```python
from build123d import *

# Parameters (mm, degrees)
SKETCH1_W           = 59.69
SKETCH1_H           = 25.4
BOSS_EXTRUDE1_DEPTH = 25.4
SKETCH2_W           = 15.24
SKETCH2_H           = 25.4
CUT_EXTRUDE1_DEPTH  = 19.05
SKETCH3_R           = 3.175
CUT_EXTRUDE2_DEPTH  = 67.101029493
SKETCH5_W           = 110.49
SKETCH5_H           = 25.4
BOSS_EXTRUDE2_DEPTH = 7.62
CUT_EXTRUDE4_DEPTH  = 92.095392309
CUT_EXTRUDE5_DEPTH  = 70.191693408
FILLET2_R           = 5.08
FILLET3_R           = 2.54


with BuildPart() as part:
    # Sketch1 → Boss-Extrude1 (new body)
    with BuildSketch(Plane(origin=(0, 0, 0), x_dir=(1, 0, 0), z_dir=(0, 1, 0))):
        Rectangle(SKETCH1_W, SKETCH1_H)
    extrude(amount=BOSS_EXTRUDE1_DEPTH)

    # Sketch2 → Cut-Extrude1 (cut)
    with BuildSketch(Plane(origin=(0, 25.4, 0), x_dir=(1, 0, 0), z_dir=(0, 1, 0))):
        Rectangle(SKETCH2_W, SKETCH2_H)
    extrude(amount=-CUT_EXTRUDE1_DEPTH, mode=Mode.SUBTRACT)

    # Sketch3 → Cut-Extrude2 (cut, through all)
    with BuildSketch(Plane.ZY.offset(29.845)):
        with Locations((0, 17.78)):
            Circle(SKETCH3_R)
    extrude(amount=-CUT_EXTRUDE2_DEPTH, mode=Mode.SUBTRACT)

    # Sketch5 → Boss-Extrude2 (add)
    with BuildSketch(Plane(origin=(0, 0, -12.7), x_dir=(-1, 0, 0), z_dir=(0, 0, -1))):
        with Locations((0, 12.7)):
            Rectangle(SKETCH5_W, SKETCH5_H)
    extrude(amount=BOSS_EXTRUDE2_DEPTH)

    # Sketch4 → Cut-Extrude4 (cut, through all)
    with BuildSketch(Plane(origin=(29.845, 0, 0), x_dir=(0, 0, -1), z_dir=(1, 0, 0))):
        with BuildLine():
            Line((-12.7, 6.35), (-12.7, 25.4))
            Line((-12.7, 25.4), (0, 25.4))
            add(Edge.make_bspline(
                [(-12.7, 6.35), (-6.35, 25.4), (0, 25.4)],
                knots=[0, 0, 0, 0.5, 0.5, 0.5], degree=2))
        make_face()
    extrude(amount=-CUT_EXTRUDE4_DEPTH, mode=Mode.SUBTRACT)

    # Sketch6 → Cut-Extrude5 (cut, through all)
    with BuildSketch(Plane(origin=(0, 0, -20.32), x_dir=(-1, 0, 0), z_dir=(0, 0, -1))):
        with BuildLine():
            Line((-44.37743079, 17.921542216), (-35.56, 17.921542216))
            ThreePointArc((-35.56, 17.921542216), (-29.939868166, 14.732), (-35.56, 11.542457784))
            Line((-35.56, 11.542457784), (-44.37743079, 11.542457784))
            ThreePointArc((-44.37743079, 11.542457784), (-47.566973006, 14.732), (-44.37743079, 17.921542216))
        make_face()
        with BuildLine():
            Line((35.56, 17.994815174), (45.556129925, 17.994815174))
            ThreePointArc((45.556129925, 17.994815174), (48.818945099, 14.732), (45.556129925, 11.469184826))
            Line((45.556129925, 11.469184826), (35.56, 11.469184826))
            ThreePointArc((35.56, 11.469184826), (29.876774509, 14.732), (35.56, 17.994815174))
        make_face()
    extrude(amount=-CUT_EXTRUDE5_DEPTH, mode=Mode.SUBTRACT)

    # Fillet2
    fillet2_edges = [part.edges().sort_by_distance(p)[0] for p in [
        (42.545, 0, -12.7),
        (-42.545, 0, -12.7),
        (29.845, 0, 0),
        (-29.845, 0, 0),
    ]]
    fillet(fillet2_edges, radius=FILLET2_R)

    # Fillet3
    fillet3_edges = [part.edges().sort_by_distance(p)[0] for p in [
        (0, 6.35, -12.7),
    ]]
    fillet(fillet3_edges, radius=FILLET3_R)


solid = part.part
```
The listing builds one solid part. Answer for the finished solid, in the listing's coordinates (mm). A direction names the side the tool comes from. Give positions to 0.01 mm unless a question says otherwise; leave off trailing zeros. Write each loop counter-clockwise with the first axis right and the second up, starting at its lowest first coordinate (ties: lowest second). Pieces come first, ordered by that corner, then holes. Notation, with made-up numbers: (60, 66) -> (101, 66) arc R15 cw to (101, 70) -> close; hole circle Ø2 at (14.5, 63). An arc over 180 degrees is marked (long way). Use one line per item in the form item = value.
1) Section A-A on z = -6.5 is taken. Write down the section's boundary in (x, y) (3 decimals), plus the area to 3 significant figures.
Result:
outline = (-29.845, 5.08) arc R5.08 ccw to (-24.765, 0) -> (24.765, 0) arc R5.08 ccw to (29.845, 5.08) -> (29.845, 25.4) -> (7.62, 25.4) -> (7.62, 6.35) -> (-7.62, 6.35) -> (-7.62, 25.4) -> (-29.845, 25.4) -> close
area = 1,210 mm²
2) Straight lines are drawn through the part: probe 1 along X at (y, z) = (6.5, 6.5) (3 decimals); probe 2 along Y at (x, z) = (-17, 0) (3 decimals); probe 3 along Z at (x, y) = (47.5, 20.25). For each, find the intervals that lie inside material, in ascending order.
Result:
probe_1 = -29.845 to -7.62, 7.62 to 29.845
probe_2 = 0 to 14.605, 20.955 to 25.4
probe_3 = -20.32 to -12.7
3) Section B-B on x = -5 is taken. Write down the section's boundary in (y, z).
Result:
outline = (0, -20.32) -> (25.4, -20.32) -> (25.4, -12.7) -> (8.89, -12.7) arc R2.54 cw to (6.35, -10.16) -> (6.35, 12.7) -> (0, 12.7) -> close
4) Section C-C on y = 16 is taken. Count the separate pieces of the cut face and the enclosed holes in it, plus the area to 3 significant figures.
Result:
separate_pieces = 5
enclosed_holes = 0
area = 1,300 mm²
5) For a pull along Y with two mould halves and no side action, classify faces 1 (the cylindrical face through (-18.89, 14.68, -0.69)), 2 (the cylindrical face through (0.107, 7.114, -11.976)), 3 (the flat face through (29.845, 15, -3)) as +Y half, -Y half, draft (parallel to the pull), parting line (faces both ways), or undercut.
Result:
face_1 = undercut
face_2 = +Y half
face_3 = draft
6) A tool of negligible diameter and unlimited length cuts with its end or side. For faces 4 (the flat face through (40, 11.542, -17)), 5 (the cylindrical face through (28.32, 1.45, -2.75)), 6 (the flat face through (-7.62, 14, -3)), 7 (the cylindrical face through (-28.32, 1.45, -2.75)), from which of +Z, -Z, +X, -X, +Y, -Y can it reach the whole face along a straight path? Write none if from no direction.
Result:
face_4 = +Z, -Z
face_5 = +Z, +X, -Y
face_6 = +Z, +Y
face_7 = +Z, -X, -Y
7) Each of these flat-tipped pins is pushed along its axis until it touches: P1, Ø5.5, axis at y = 17.78, z = 0, coming from the -X side; P2, Ø5, axis at x = 31.5, z = -5, coming from the -Y side; P3, Ø8, axis at x = 34, z = -11, coming from the -Y side; P4, Ø7.5, axis at x = 3.5, y = 20.5, coming from the +Z side. Where does it stop, or does it pass through?
Result:
P1 = through
P2 = 2.27
P3 = 0.83
P4 = -12.7
